The listing builds one solid part. Answer for the finished solid, in the listing's coordinates (mm). Face numbers are marked on the shaded views. A direction names the side the tool comes from. Round coordinates to 2 decimals unless told otherwise and drop trailing zeros. Write each question's results on one line, items separated by ' | '. Start each with the question number.
```python
from build123d import *

# Parameters (mm, degrees)
ESQUISSE1_R                          = 38.1
BOSS_EXTRU_1_DEPTH                   = 27
ESQUISSE3_R                          = 25.4
ENL_V_MAT_EXTRU_2_DEPTH              = 24
ESQUISSE5_R                          = 11
ENL_V_MAT_EXTRU_3_DEPTH              = 3
ESQUISSE8_R                          = 38.1
ESQUISSE8_R_2                        = 34.925
ENL_V_MAT_EXTRU_5_DEPTH              = 2
R_P_TITION_LIN_AIRE1_COUNT           = 6
R_P_TITION_LIN_AIRE1_PITCH           = 4
D_GAGEMENT_61_D                      = 3.7973
F_1_8_0_126_TROUS_DE_CENTRAGE1_D     = 3.2004
F_1_8_0_126_TROUS_DE_CENTRAGE1_DEPTH = 27
F_1_8_0_126_TROUS_DE_CENTRAGE1_TIP   = 0.961497163


with BuildPart() as part:
    # Esquisse1 → Boss.-Extru.1 (new body)
    with BuildSketch(Plane.XY):
        with Locations((23.679503876, 29.670703652)):
            Circle(ESQUISSE1_R)
    extrude(amount=BOSS_EXTRU_1_DEPTH)

    # Esquisse3 → Enlèv. mat.-Extru.2 (cut)
    with BuildSketch(Plane.XY.offset(27)):
        with Locations((23.679503876, 29.670703652)):
            Circle(ESQUISSE3_R)
    extrude(amount=-ENL_V_MAT_EXTRU_2_DEPTH, mode=Mode.SUBTRACT)

    # Esquisse5 → Enlèv. mat.-Extru.3 (cut)
    with BuildSketch(Plane(origin=(0, 0, 0), x_dir=(-1, 0, 0), z_dir=(0, 0, -1))):
        with Locations((-23.679503876, 29.670703652)):
            Circle(ESQUISSE5_R)
    extrude(amount=-ENL_V_MAT_EXTRU_3_DEPTH, mode=Mode.SUBTRACT)

    # Esquisse8 → Enlèv. mat.-Extru.5 (cut)
    with BuildSketch(Plane.XY.offset(27)):
        with Locations((23.679503876, 29.670703652)):
            Circle(ESQUISSE8_R)
        with Locations((23.679503876, 29.670703652)):
            Circle(ESQUISSE8_R_2, mode=Mode.SUBTRACT)
    enl_v_mat_extru_5 = extrude(amount=-ENL_V_MAT_EXTRU_5_DEPTH, mode=Mode.SUBTRACT)

    # Répétition linéaire1: Enlèv. mat.-Extru.5 ×6
    with Locations(*[(0, 0, -i * R_P_TITION_LIN_AIRE1_PITCH) for i in range(1, R_P_TITION_LIN_AIRE1_COUNT)]):
        add(enl_v_mat_extru_5, mode=Mode.SUBTRACT)

    # Dégagement #61 (through all)
    with Locations(Plane(origin=(0, 0, 0), x_dir=(-1, 0, 0), z_dir=(0, 0, -1))):
        with Locations((-38.760753876, 55.792194893), (6.482996124, 29.670703652), (-38.760753876, 3.54921241)):
            Hole(D_GAGEMENT_61_D / 2)

    # 1/8 (0.126) Trous de centrage1
    with Locations(Plane(origin=(0, 0, 0), x_dir=(-1, 0, 0), z_dir=(0, 0, -1))):
        with Locations((-23.679503876, 61.420703652), (-12.820364325, -0.164537058)):
            Hole(F_1_8_0_126_TROUS_DE_CENTRAGE1_D / 2, depth=F_1_8_0_126_TROUS_DE_CENTRAGE1_DEPTH)
            with Locations((0, 0, -(F_1_8_0_126_TROUS_DE_CENTRAGE1_DEPTH + F_1_8_0_126_TROUS_DE_CENTRAGE1_TIP / 2))):  # 118° drill point
                Cone(0, F_1_8_0_126_TROUS_DE_CENTRAGE1_D / 2, F_1_8_0_126_TROUS_DE_CENTRAGE1_TIP, mode=Mode.SUBTRACT)


solid = part.part
```
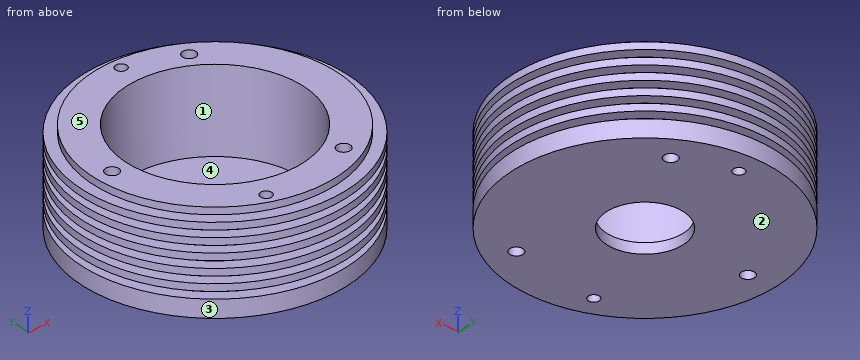
Q1. The part is cut by section A-A, the plane x = 39. State how many separate pieces and enclosed holes the cut face has, then the cut area to 3 significant figures.
Q2. For the marked faces 1 and 2, determine the directions among +Z, -Z, +X, -X, +Y, -Y from which every point of the face is accessible in a straight line to the end or side of a thin tool.
Q3. Each of these flat-tipped pins is pushed along its axis until it touches: pin 1 (5 mm diameter, centred on x = 51.5, y = 50.5, fed in from -Z); pin 2 (2 mm diameter, centred on y = 51, z = 23.5, fed in from -X); pin 3 (3 mm diameter, centred on y = 5, z = 8, fed in from -X) (3 decimals); pin 4 (5 mm diameter, centred on x = 2, z = 13.5, fed in from -Y). Where does it stop, or does it pass through?
Q4. Find the intervals of material crossed by line 1 (Z direction, x = 43, y = 61.5); line 2 (Y direction, x = 12.5, z = 4); line 3 (Z direction, x = 13.5, y = 48.5), in increasing order.
Q5. Determine the mould class of the marked faces 3, 4 and 5 for opening direction Y: pulls with the +Y half, pulls with the -Y half, needs draft (parallel to the pull), parting line crosses it, or undercut.
Answers follow:
1) separate pieces: 3 | enclosed holes: 0 | area: 624 mm^2
2) face 1: +Z | face 2: -Z, +X, -X, +Y, -Y
3) pin 1: z = 0 | pin 2: x = -8.54 | pin 3: x = -6.565 | pin 4: y = -3.22
4) line 1: 0 to 5, 7 to 9, 11 to 13, 15 to 17, 19 to 21, 23 to 25 | line 2: -6.75 to -1.73, 1.4 to 6.86, 52.48 to 66.09 | line 3: 0 to 3
5) face 3: parting line crosses it | face 4: undercut | face 5: needs draft
